Geometry check sheet. Reference: the model listing, model coordinates, mm. Coordinates: 2 decimals unless noted, no trailing zeros. Loops run counter-clockwise (first coordinate to the right, second up) from the corner with the lowest first, then second, coordinate; pieces in that order, holes last.
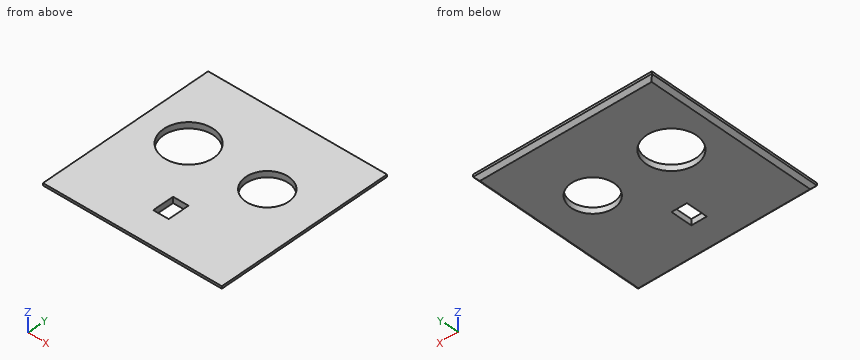
from build123d import *

# Parameters (mm, degrees)
SKETCH002_R      = 21
SKETCH002_R_2    = 18
SKETCH002_W      = 13
SKETCH002_H      = 18
EXTRUDE002_DEPTH = 10
BOX002_W         = 150
BOX002_H         = 150
BOX002_DEPTH     = 5
CHAMFER_SIZE     = 3


with BuildPart() as extrude002:
    # Sketch002 (on Face6 of Box002) → Extrude002 (new body)
    with BuildSketch(Plane.XY.offset(5)):
        with Locations((39.413204, 89.551971)):
            Circle(SKETCH002_R)
        with Locations((105.700333, 89.247101)):
            Circle(SKETCH002_R_2)
        with Locations((74.540915, 35.410171)):
            Rectangle(SKETCH002_W, SKETCH002_H)
    extrude(amount=EXTRUDE002_DEPTH)


with BuildPart() as extrude002_1:
    # Extrude002 placement: moved
    add(extrude002.part.moved(Location((0, 0, -7))))


with BuildPart() as tapacaja003:
    # Box002 → Box002 (new body)
    with BuildSketch(Plane.XY):
        with Locations((75, 75)):
            Rectangle(BOX002_W, BOX002_H)
    extrude(amount=BOX002_DEPTH)

    # Cut002: cut Extrude002
    add(extrude002_1.part, mode=Mode.SUBTRACT)


with BuildPart() as tapacaja003_1:
    # Cut002 placement: moved
    add(tapacaja003.part.moved(Location((0, 0, 61))))

    # Chamfer
    chamfer_edges = [tapacaja003_1.edges().sort_by_distance(p)[0] for p in [
        (0, 75, 61),
        (75, 0, 61),
        (75, 150, 61),
        (150, 75, 61),
    ]]
    chamfer(chamfer_edges, length=CHAMFER_SIZE)


with BuildPart() as tapacaja003_2:
    # Chamfer placement: moved
    add(tapacaja003_1.part.moved(Location((0, 0, -4))))


solid = tapacaja003_2.part
(1) Sectioned sample at A-A on y = 31.5. Record the cut outline in (x, z), and give its area (3 significant figures).
Findings:
outline: (0, 60) - (3, 57) - (68.04, 57) - (68.04, 62) - (0, 62) - close; (81.04, 57) - (147, 57) - (150, 60) - (150, 62) - (81.04, 62) - close
area: 676 mm2
(2) Sectioned sample at D-D on z = 58.7. Record the cut outline in (x, y).
Findings:
outline: (1.3, 1.3) - (148.7, 1.3) - (148.7, 148.7) - (1.3, 148.7) - close; hole circle Ø42 at (39.41, 89.55); hole (68.04, 26.41) - (81.04, 26.41) - (81.04, 44.41) - (68.04, 44.41) - close; hole circle Ø36 at (105.7, 89.25)
(3) Sectioned sample at C-C on y = 77. Record the cut outline in (x, z).
Findings:
outline: (0, 60) - (3, 57) - (22.58, 57) - (22.58, 62) - (0, 62) - close; (56.25, 57) - (92.51, 57) - (92.51, 62) - (56.25, 62) - close; (118.89, 57) - (147, 57) - (150, 60) - (150, 62) - (118.89, 62) - close
(4) Sectioned sample at B-B on x = 99.5. Record the cut outline in (y, z).
Findings:
outline: (0, 60) - (3, 57) - (72.35, 57) - (72.35, 62) - (0, 62) - close; (106.15, 57) - (147, 57) - (150, 60) - (150, 62) - (106.15, 62) - close
(5) Scan lines: L1, parallel to X at y = 101, z = 58.25; L2, parallel to Y at x = 74, z = 60.15; L3, parallel to X at y = 96.5, z = 59.9. Record each from-to range of solid material in increasing order.
Findings:
L1: x = 1.75 to 21.81, 57.02 to 92.07, 119.33 to 148.25
L2: y = 0 to 26.41, 44.41 to 150
L3: x = 0.1 to 19.6, 59.23 to 89.23, 122.17 to 149.9
(6) Gauge pin test, flat end, axial feed: pin 1 Ø2 at (y, z) = (103.5, 58.5) entering from +X. Record the tip position at first contact, or that the pin passes through.
Findings:
pin 1: stops at x = 149.5
